For this review, use the dimensioned drawing (mm, ordinates from the lowest corner) and the shaded views. A direction names the side the tool comes from. Give positions to 0.01 mm unless a question says otherwise; leave off trailing zeros. Order: outer loops, then holes, each group sorted by start corner. A loop starts at its lowest first (then second) coordinate and runs counter-clockwise, first axis right, second up.
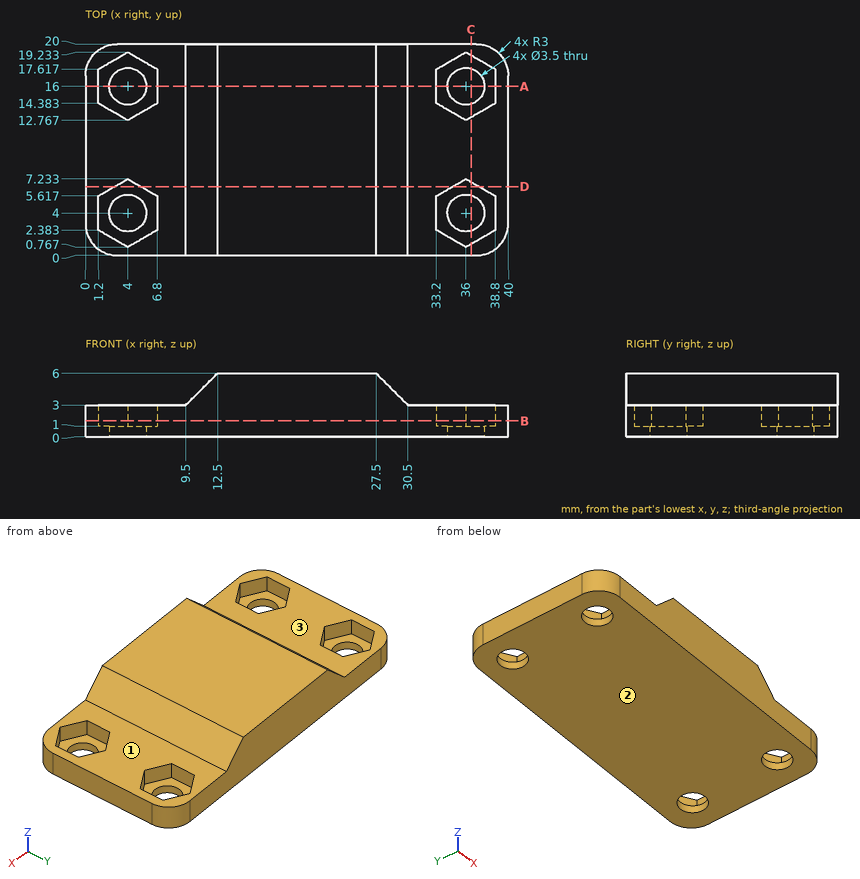
1. Take a section at A-A (y = 16). State the section outline as (x, z) points, then the cut area to 3 significant figures.
Recorded:
outline: (0, 0) - (2.25, 0) - (2.25, 1) - (1.2, 1) - (1.2, 3) - (0, 3) - close; (5.75, 0) - (34.25, 0) - (34.25, 1) - (33.2, 1) - (33.2, 3) - (30.5, 3) - (27.5, 6) - (12.5, 6) - (9.5, 3) - (6.8, 3) - (6.8, 1) - (5.75, 1) - close; (37.75, 0) - (40, 0) - (40, 3) - (38.8, 3) - (38.8, 1) - (37.75, 1) - close
area: 145 mm2
2. Take a section at D-D (y = 6.5). State the section outline as (x, z) points.
Recorded:
outline: (0, 0) - (40, 0) - (40, 3) - (37.27, 3) - (37.27, 1) - (34.73, 1) - (34.73, 3) - (30.5, 3) - (27.5, 6) - (12.5, 6) - (9.5, 3) - (5.27, 3) - (5.27, 1) - (2.73, 1) - (2.73, 3) - (0, 3) - close
3. Take a section at B-B (z = 1.5). State how many separate pieces and enclosed holes the cut face has.
Recorded:
separate pieces: 1
enclosed holes: 4
4. Take a section at C-C (x = 36.5). State the section outline as (y, z) points (1 decimal).
Recorded:
outline: (0, 0) - (2.3, 0) - (2.3, 1) - (1.1, 1) - (1.1, 3) - (0, 3) - close; (5.7, 0) - (14.3, 0) - (14.3, 1) - (13.1, 1) - (13.1, 3) - (6.9, 3) - (6.9, 1) - (5.7, 1) - close; (17.7, 0) - (20, 0) - (20, 3) - (18.9, 3) - (18.9, 1) - (17.7, 1) - close
5. Machinability: for the marked faces 1, 2 and 3, which of the approach directions +Z, -Z, +X, -X, +Y, -Y give a long, thin tool a straight path to every point of the face, cutting with its end or side? Answer none if there is none.
Recorded:
face 1: +Z, +X, +Y, -Y
face 2: -Z, +X, -X, +Y, -Y
face 3: +Z, -X, +Y, -Y
6. For pin 1 (3 mm diameter, centred on x = 36, y = 15, fed in from +Z), flat-tipped, find the tip position at first contact; note if it passes through.
Recorded:
pin 1: stops at z = 1
7. For line 1 along Y through (x, z) = (4, 0.4); line 2 along X through (y, z) = (16, 0.45); line 3 along Y through (x, z) = (37, 1.9) (1 decimal), list the stretches that pass through material, from the lowest coordinate up.
Recorded:
line 1: y = 0 to 2.25, 5.75 to 14.25, 17.75 to 20
line 2: x = 0 to 2.25, 5.75 to 34.25, 37.75 to 40
line 3: y = 0 to 1.3, 6.7 to 13.3, 18.7 to 20
